Read the model definition and answer for the solid it produces. Units are mm, in the model's axes. Give positions to 0.01 mm unless a question says otherwise; leave off trailing zeros. Write each loop counter-clockwise with the first axis right and the second up, starting at its lowest first coordinate (ties: lowest second). Pieces come first, ordered by that corner, then holes. Notation, with made-up numbers: M 41,52 L 57,52 A23 cw 57,71 Z; hole C 27.25,6 d3. An arc over 180 degrees is marked long. Use a Markdown table: item, result. Add a question column.
Item 1: Given P1, Ø9, axis at x = 22.5, z = 210.5, coming from the -Y side; P2, Ø9, axis at x = 499.5, y = 87.5, coming from the +Z side, each flat-ended and moving along its own axis, determine where each tip first touches the part or whether it passes through.
Item 2: A cutting plane is placed at C-C on y = 36.5. Determine the outline of the cut face in (x, z).
Item 3: A cutting plane is placed at A-A on x = 40. Determine the outline of the cut face in (y, z).
Item 4: Consider probe 1 along Y at (x, z) = (223, 13); probe 2 along X at (y, z) = (18.5, 184); probe 3 along Z at (x, y) = (475, 24.5). Determine where each line is inside the solid, lowest interval first. Write a range as [from, to].
Item 5: A cutting plane is placed at B-B on z = 167. Determine the outline of the cut face in (x, y).
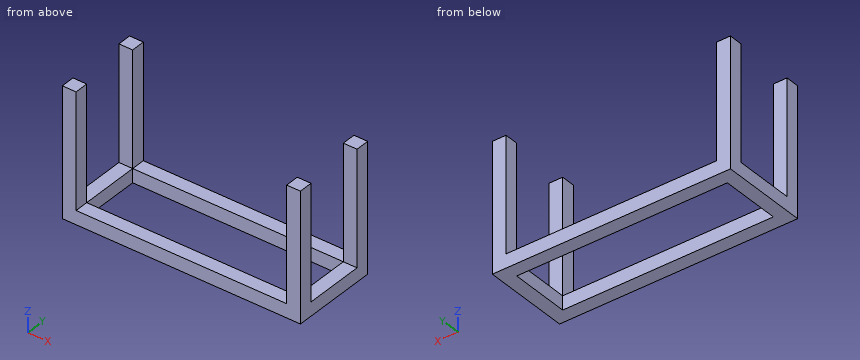
from build123d import *

# Parameters (mm, degrees)
SKETCH_1_W      = 30
SKETCH_1_H      = 190
SKETCH_1_W_2    = 460
SKETCH_1_H_2    = 30
EXTRUDE_1_DEPTH = 30
SKETCH_2_W      = 30
SKETCH_2_H      = 30
EXTRUDE_2_DEPTH = 250


with BuildPart() as part:
    # 草图1 → 凸台-拉伸1 (new body)
    with BuildSketch(Plane.XY):
        with Locations((15, 95)):
            Rectangle(SKETCH_1_W, SKETCH_1_H)
        with Locations((260, 175)):
            Rectangle(SKETCH_1_W_2, SKETCH_1_H_2)
        with Locations((260, 15)):
            Rectangle(SKETCH_1_W_2, SKETCH_1_H_2)
        Polygon((490, 30), (490, 0), (520, 0), (520, 190), (490, 190), (490, 160), align=None)
    extrude(amount=EXTRUDE_1_DEPTH)

    # 草图2 → 凸台-拉伸2 (add)
    with BuildSketch(Plane.XY.offset(30)):
        with Locations((15, 175)):
            Rectangle(SKETCH_2_W, SKETCH_2_H)
        with Locations((15, 15)):
            Rectangle(SKETCH_2_W, SKETCH_2_H)
        with Locations((505, 175)):
            Rectangle(SKETCH_2_W, SKETCH_2_H)
        with Locations((505, 15)):
            Rectangle(SKETCH_2_W, SKETCH_2_H)
    extrude(amount=EXTRUDE_2_DEPTH)


solid = part.part
Filled in:
| question | item | result |
|---|---|---|
| 1 | P1 | y = 0 |
| 1 | P2 | z = 30 |
| 2 | outline | M 0,0 L 30,0 L 30,30 L 0,30 Z; M 490,0 L 520,0 L 520,30 L 490,30 Z |
| 3 | outline | M 0,0 L 30,0 L 30,30 L 0,30 Z; M 160,0 L 190,0 L 190,30 L 160,30 Z |
| 4 | probe 1 | [0, 30], [160, 190] |
| 4 | probe 2 | [0, 30], [490, 520] |
| 4 | probe 3 | [0, 30] |
| 5 | outline | M 0,0 L 30,0 L 30,30 L 0,30 Z; M 0,160 L 30,160 L 30,190 L 0,190 Z; M 490,0 L 520,0 L 520,30 L 490,30 Z; M 490,160 L 520,160 L 520,190 L 490,190 Z |
